Input: part model. Units: mm. Frame: model coordinates. Round coordinates to 2 decimals unless told otherwise and drop trailing zeros. Loops run counter-clockwise (first coordinate to the right, second up) from the corner with the lowest first, then second, coordinate; pieces in that order, holes last. Notation, with made-up numbers: (-18, -22) - (31, -22) arc R34 cw to (31, 12) - close; hole circle Ø6 at (85, 0.25). An arc over 180 degrees is marked (long way). One line per question, with ' | ' between items. Start each with the question number.
from build123d import *

# Parameters (mm, degrees)
SKETCH1_W          = 6.35
SKETCH1_H          = 36.5125
BASE_FLANGE1_DEPTH = 19.05
CUT_EXTRUDE1_REACH = 29.139
CUT_EXTRUDE2_REACH = 29.139
SKETCH4_R          = 4.365625
SKETCH4_R_2        = 1.9558
SKETCH4_R_3        = 3.9751
FILLET1_R          = 6.35
FILLET2_R          = 3.175


# Sheet-metal steps are written as plain solids
with BuildPart() as part:
    # Sketch1 → Base-Flange1 (new, symmetric)
    with BuildSketch(Plane(origin=(0, 0, 0), x_dir=(0, 0, -1), z_dir=(1, 0, 0))):
        with Locations((-3.175, 0)):
            Rectangle(SKETCH1_W, SKETCH1_H)
    extrude(amount=BASE_FLANGE1_DEPTH, both=True)

    # Sketch3 → Cut-Extrude1 (cut, up to next)
    with BuildSketch(Plane.XY.offset(6.35), mode=Mode.PRIVATE) as cut_extrude1_sk1:
        Polygon((-19.05, 18.25625), (-19.05, -18.25625), (-17.455829822, 18.25625), align=None)
    cut_extrude1_tool1 = extrude(cut_extrude1_sk1.sketch, amount=-CUT_EXTRUDE1_REACH, mode=Mode.PRIVATE) & part.part
    # Sketch3 → Cut-Extrude1 (cut, up to next)
    with BuildSketch(Plane.XY.offset(6.35), mode=Mode.PRIVATE) as cut_extrude1_sk2:
        Polygon((19.05, 18.25625), (19.05, -10.31875), (-9.525, 18.25625), align=None)
    cut_extrude1_tool2 = extrude(cut_extrude1_sk2.sketch, amount=-CUT_EXTRUDE1_REACH, mode=Mode.PRIVATE) & part.part
    add(cut_extrude1_tool1.solids().sort_by_distance((-18.51861, 6.085417, 6.35))[0], mode=Mode.SUBTRACT)
    add(cut_extrude1_tool2.solids().sort_by_distance((9.525, 8.73125, 6.35))[0], mode=Mode.SUBTRACT)

    # Sketch4 → Cut-Extrude2 (cut, up to next)
    with BuildSketch(Plane.XY.offset(6.35), mode=Mode.PRIVATE) as cut_extrude2_sk1:
        with Locations((-11.1125, -11.90625)):
            Circle(SKETCH4_R)
    cut_extrude2_tool1 = extrude(cut_extrude2_sk1.sketch, amount=-CUT_EXTRUDE2_REACH, mode=Mode.PRIVATE) & part.part
    # Sketch4 → Cut-Extrude2 (cut, up to next)
    with BuildSketch(Plane.XY.offset(6.35), mode=Mode.PRIVATE) as cut_extrude2_sk2:
        with Locations((14.2875, -11.90625)):
            Circle(SKETCH4_R_2)
    cut_extrude2_tool2 = extrude(cut_extrude2_sk2.sketch, amount=-CUT_EXTRUDE2_REACH, mode=Mode.PRIVATE) & part.part
    # Sketch4 → Cut-Extrude2 (cut, up to next)
    with BuildSketch(Plane.XY.offset(6.35), mode=Mode.PRIVATE) as cut_extrude2_sk3:
        with Locations((-11.1125, 10.31875)):
            Circle(SKETCH4_R_3)
    cut_extrude2_tool3 = extrude(cut_extrude2_sk3.sketch, amount=-CUT_EXTRUDE2_REACH, mode=Mode.PRIVATE) & part.part
    add(cut_extrude2_tool1.solids().sort_by_distance((-11.1125, -11.90625, 6.35))[0], mode=Mode.SUBTRACT)
    add(cut_extrude2_tool2.solids().sort_by_distance((14.2875, -11.90625, 6.35))[0], mode=Mode.SUBTRACT)
    add(cut_extrude2_tool3.solids().sort_by_distance((-11.1125, 10.31875, 6.35))[0], mode=Mode.SUBTRACT)

    # Fillet1
    fillet1_edges = [part.edges().sort_by_distance(p)[0] for p in [
        (-17.455829822, 18.25625, 3.175),
    ]]
    fillet(fillet1_edges, radius=FILLET1_R)

    # Fillet2
    fillet2_edges = [part.edges().sort_by_distance(p)[0] for p in [
        (-9.525, 18.25625, 3.175),
    ]]
    fillet(fillet2_edges, radius=FILLET2_R)


solid = part.part
(1) Section B-B, the plane x = -13. Output: boundary loops of the cut face in (y, z).
(2) Pin query (flat end, axial travel): P1, Ø2, axis at y = 5.5, z = 5.5, coming from the +X side; P2, Ø1.5, axis at y = 1.5, z = 3.5, coming from the -X side. Return the tip coordinate at first contact, or that it passes through.
(3) Section C-C, the plane z = 2. Give the number of separate pieces and of enclosed holes in the cut face, plus the area to 3 significant figures.
(4) Line query: line 1 along X through (y, z) = (-11, 1.25); line 2 along Y through (x, z) = (-10, 2) (1 decimal); line 3 along Y through (x, z) = (12.5, 4.5). Output: solid intervals per line, ascending. Write a range as from..to.
(5) Pull-direction query (Y, two-part tool) for faces 1 (the face through (-9.64, 18.02, 3.13)), 2 (the face through (19.05, -14, 3)), 3 (the face through (-7.08, -13.58, 3.22)), 4 (the face through (-8.976, 13.671, 3.219)); classes: released by +Y, released by -Y, zero draft, split by the parting line, or undercut.
(6) Section D-D, the plane y = 11. Output: boundary loops of the cut face in (x, z), plus the area to 3 significant figures.
(7) Section A-A, the plane y = -14.5. Output: boundary loops of the cut face in (x, z).
Derived:
1) outline: (-18.26, 0) - (-15.84, 0) - (-15.84, 6.35) - (-18.26, 6.35) - close; (-7.97, 0) - (6.82, 0) - (6.82, 6.35) - (-7.97, 6.35) - close; (13.82, 0) - (18.05, 0) - (18.05, 6.35) - (13.82, 6.35) - close
2) P1: stops at x = 4.23 | P2: stops at x = -18.22
3) separate pieces: 1 | enclosed holes: 3 | area: 824 mm²
4) line 1: x = -18.73..-15.38, -6.84..12.55, 16.02..19.05 | line 2: y = -18.3..-16.1, -7.7..6.5, 14.1..18.1 | line 3: y = -18.26..-12.7, -11.11..-3.77
5) face 1: released by +Y | face 2: zero draft | face 3: undercut | face 4: undercut
6) outline: (-17.77, 0) - (-15.03, 0) - (-15.03, 6.35) - (-17.77, 6.35) - close; (-7.2, 0) - (-2.27, 0) - (-2.27, 6.35) - (-7.2, 6.35) - close | area: 48.7 mm²
7) outline: (-18.89, 0) - (-14.62, 0) - (-14.62, 6.35) - (-18.89, 6.35) - close; (-7.6, 0) - (19.05, 0) - (19.05, 6.35) - (-7.6, 6.35) - close
